Solid Edge part; units mm, degrees
sketch "Sketch1" plane through (0, 0, 0) normal (0, 0, 1) x (1, 0, 0)
  circle A0 centre (0, 0) radius 5
extrude "Protrusion1" add sketch "Sketch1" along normal blind 6
sketch "Sketch2" plane through (0, 0, 6) normal (0, 0, 1) x (1, 0, 0)
  circle A0 centre (0, 0) radius 2
extrude "Cutout1" cut sketch "Sketch2" against normal up to vertex (6 mm away)
fillet "Round_1" radius 2 1 edges at (-5, 0, 6)
fillet "Round_2" radius 2 1 edges at (-5, 0, 0)
Model file for the job. Use its own axes, mm. Coordinates: 2 decimals unless noted, no trailing zeros. Loops run counter-clockwise (first coordinate to the right, second up) from the corner with the lowest first, then second, coordinate; pieces in that order, holes last. Notation, with made-up numbers: (75, -36.75) -> (88, -36.75) arc R15 cw to (88, -27.75) -> close; hole circle Ø9 at (68.25, 47.5). An arc over 180 degrees is marked (long way). Answer as a JSON object with one key per item and string values.
Q1. Cut at D-D (z = 5.1). List the corners of the cut face in (x, y), and give its area (3 significant figures).
Report:
{"outline": "circle Ø9.34 at (0, 0); hole circle Ø4 at (0, 0)", "area": "56.0 mm2"}
Q2. Cut at C-C (z = 3.25). List the corners of the cut face in (x, y).
Report:
{"outline": "circle Ø10 at (0, 0); hole circle Ø4 at (0, 0)"}
Q3. Flat gauge pins, fed straight in: P1, Ø1.5, axis at y = 3, z = 3, coming from the -X side; P2, Ø4.5, axis at x = 0, y = 0, coming from the +Z side; P3, Ø2, axis at x = 3, z = 2, coming from the -Y side; P4, Ø1.5, axis at x = -3, y = 3, coming from the +Z side. Where does each tip first touch, or does it go through?
Report:
{"P1": "stops at x = -4.47", "P2": "stops at z = 6", "P3": "stops at y = -4.58", "P4": "stops at z = 5.94"}
Q4. Probe probe 1 along Y at (x, z) = (0, 3.85); probe 2 along X at (y, z) = (-0.25, 0.7); probe 3 along X at (y, z) = (0.5, 5.35). List the from-to ranges inside material, lowest first.
Report:
{"probe 1": "y = -5 to -2, 2 to 5", "probe 2": "x = -4.51 to -1.98, 1.98 to 4.51", "probe 3": "x = -4.45 to -1.94, 1.94 to 4.45"}
Q5. Cut at A-A (x = 0). List the corners of the cut face in (y, z).
Report:
{"outline": "(-5, 2) arc R2 ccw to (-3, 0) -> (-2, 0) -> (-2, 6) -> (-3, 6) arc R2 ccw to (-5, 4) -> close; (2, 0) -> (3, 0) arc R2 ccw to (5, 2) -> (5, 4) arc R2 ccw to (3, 6) -> (2, 6) -> close"}
